```python
from build123d import *

# Parameters (mm, degrees)
SKETCH_1_R          = 3.25
EXTRUDE_1_DEPTH     = 2
SKETCH_1_3_W        = 8.5
SKETCH_1_3_H        = 1.5
EXTRUDE_2_DEPTH     = 1
SKETCH_2_W          = 4
SKETCH_2_H          = 1.5
EXTRUDE_3_DEPTH     = 6.5
CUT_EXTRUDE_1_DEPTH = 13
SKETCH_4_R          = 1.2
CUT_EXTRUDE_2_DEPTH = 13
SKETCH_5_W          = 0.419062678
SKETCH_5_H          = 3
CUT_EXTRUDE_3_DEPTH = 12
SKETCH_7_W          = 3.667600517
SKETCH_7_H          = 1.5
EXTRUDE_4_DEPTH     = 18
SKETCH_8_W          = 3.667600517
SKETCH_8_H          = 5.48261061
EXTRUDE_5_DEPTH     = 9
SKETCH_9_W          = 2.616581955
SKETCH_9_H          = 4.806747763
EXTRUDE_6_DEPTH     = 9
SKETCH_10_R         = 1.719166773
CUT_EXTRUDE_4_DEPTH = 11.421628998
CUT_EXTRUDE_5_DEPTH = 13
EXTRUDE_7_DEPTH     = 8.843258


with BuildPart() as part:
    # 草图1 → 凸台-拉伸1 (new body)
    with BuildSketch(Plane(origin=(0, 0, 0), x_dir=(1, 0, 0), z_dir=(0, 1, 0))):
        Polygon((-4.25, -4.25), (-4.25, -6), (4.25, -6), (4.25, -4.25), (4.25, 4.25), (4.25, 6), (-4.25, 6), (-4.25, 4.25), align=None)
        Circle(SKETCH_1_R, mode=Mode.SUBTRACT)
    extrude(amount=EXTRUDE_1_DEPTH)

    # 草图1<3> → 凸台-拉伸2 (add)
    with BuildSketch(Plane(origin=(0, 0, 0), x_dir=(1, 0, 0), z_dir=(0, 1, 0))):
        with Locations((0, -5.25)):
            Rectangle(SKETCH_1_3_W, SKETCH_1_3_H)
        with Locations((0, 5.25)):
            Rectangle(SKETCH_1_3_W, SKETCH_1_3_H)
    extrude(amount=-EXTRUDE_2_DEPTH)

    # 草图2 → 凸台-拉伸3 (add)
    with BuildSketch(Plane.XZ.offset(1)):
        with Locations((-1.830937322, -5.25)):
            Rectangle(SKETCH_2_W, SKETCH_2_H)
        with Locations((-1.830937322, 5.25)):
            Rectangle(SKETCH_2_W, SKETCH_2_H)
    extrude(amount=EXTRUDE_3_DEPTH)

    # 草图3 → 切除-拉伸1 (cut, through all)
    with BuildSketch(Plane(origin=(0, 0, -6), x_dir=(-1, 0, 0), z_dir=(0, 0, -1))):
        Polygon((-0.169062678, -4.270246896), (0.163336805, -7.5), (-0.169062678, -7.5), align=None)
    extrude(amount=-CUT_EXTRUDE_1_DEPTH, mode=Mode.SUBTRACT)

    # 草图4 → 切除-拉伸2 (cut, through all)
    with BuildSketch(Plane(origin=(0, 0, -6), x_dir=(-1, 0, 0), z_dir=(0, 0, -1))):
        with Locations((1.920905564, -6)):
            Circle(SKETCH_4_R)
    extrude(amount=-CUT_EXTRUDE_2_DEPTH, mode=Mode.SUBTRACT)

    # 草图5 → 切除-拉伸3 (cut)
    with BuildSketch(Plane(origin=(0, 0, -6), x_dir=(-1, 0, 0), z_dir=(0, 0, -1))):
        with Locations((4.040468661, 0.5)):
            Rectangle(SKETCH_5_W, SKETCH_5_H)
    extrude(amount=-CUT_EXTRUDE_3_DEPTH, mode=Mode.SUBTRACT)

    # 草图7 → 凸台-拉伸4 (add)
    with BuildSketch(Plane.XZ.offset(7.5)):
        with Locations((-1.997137064, 5.25)):
            Rectangle(SKETCH_7_W, SKETCH_7_H)
        with Locations((-1.997137064, -5.25)):
            Rectangle(SKETCH_7_W, SKETCH_7_H)
    extrude(amount=EXTRUDE_4_DEPTH)

    # 草图8 → 凸台-拉伸5 (add)
    with BuildSketch(Plane(origin=(0, 0, 4.5), x_dir=(-1, 0, 0), z_dir=(0, 0, -1))):
        with Locations((1.997137064, -22.758694695)):
            Rectangle(SKETCH_8_W, SKETCH_8_H)
    extrude(amount=EXTRUDE_5_DEPTH)

    # 草图9 → 凸台-拉伸6 (add)
    with BuildSketch(Plane(origin=(-0.163336805, 0, 0), x_dir=(0, 0, -1), z_dir=(1, 0, 0))):
        with Locations((3.113338021, -22.793424654)):
            Rectangle(SKETCH_9_W, SKETCH_9_H)
        with Locations((-3.113338021, -22.793424654)):
            Rectangle(SKETCH_9_W, SKETCH_9_H)
    extrude(amount=EXTRUDE_6_DEPTH)

    # 草图10 → 切除-拉伸4 (cut, through all)
    with BuildSketch(Plane(origin=(0, 0, -4.421628998), x_dir=(-1, 0, 0), z_dir=(0, 0, -1))):
        with Locations((-5.836663195, -22.894386417)):
            Circle(SKETCH_10_R)
    extrude(amount=-CUT_EXTRUDE_4_DEPTH, mode=Mode.SUBTRACT)

    # 草图11 → 切除-拉伸5 (cut, through all)
    with BuildSketch(Plane(origin=(0, 0, -6), x_dir=(-1, 0, 0), z_dir=(0, 0, -1))):
        Polygon((3.830937322, -22.440555736), (-3.067140817, -25.196798535), (0.381898253, -26.676483331), (3.830937322, -26.676483331), align=None)
    extrude(amount=-CUT_EXTRUDE_5_DEPTH, mode=Mode.SUBTRACT)

    # 草图13 → 凸台-拉伸7 (add)
    with BuildSketch(Plane(origin=(0, 0, -4.421628998), x_dir=(-1, 0, 0), z_dir=(0, 0, -1))):
        Polygon((-2.471529716, -20.390050772), (3.830937322, -16.84684298), (3.830937322, -20.390050772), align=None)
    extrude(amount=-EXTRUDE_7_DEPTH)


solid = part.part
```
Check sheet for the modelled part. Datum: model origin and axes. Units: mm. A direction names the side the tool comes from. Round coordinates to 2 decimals unless told otherwise and drop trailing zeros. Loops run counter-clockwise (first coordinate to the right, second up) from the corner with the lowest first, then second, coordinate; pieces in that order, holes last. Notation, with made-up numbers: M 27.5,60 L 43.5,60 A19 ccw 43.5,95 Z; hole C 16,-7 d5. An arc over 180 degrees is marked long. Answer as a JSON object with one key per item and string values.
1. Mould release check, pull along Z, two halves, no side actions. Record for faces 1 (the flat face through (0, -5.9, -5.3)), 2 (the flat face through (-2, -10, 4.5)), 3 (the flat face through (-2, -8, -6)): pulls with the +Z half, pulls with the -Z half, needs draft (parallel to the pull), parting line crosses it, or undercut.
Reply:
{"face 1": "needs draft", "face 2": "undercut", "face 3": "pulls with the -Z half"}
2. Section check B-B (x = 1.5). Record the boundary of the cut face in (y, z), plus the area to 3 significant figures.
Reply:
{"outline": "M -24.57,-4.42 L -19.84,-4.42 L -19.84,4.42 L -24.57,4.42 L -24.57,1.81 L -20.39,1.81 L -20.39,-1.81 L -24.57,-1.81 Z; M -1,-6 L 2,-6 L 2,-2.88 L 0,-2.88 L 0,-4.5 L -1,-4.5 Z; M -1,4.5 L 0,4.5 L 0,2.88 L 2,2.88 L 2,6 L -1,6 Z", "area": "42.2 mm²"}
3. Section check C-C (y = -0.5). Record the boundary of the cut face in (x, z).
Reply:
{"outline": "M -3.83,-6 L 4.25,-6 L 4.25,-4.5 L -3.83,-4.5 Z; M -3.83,4.5 L 4.25,4.5 L 4.25,6 L -3.83,6 Z"}
4. Access from +Z, -Z, +X, -X, +Y, -Y to the whole of each face (thin tool, end or side, straight path). Record for faces 4 (the flat face through (2, -22, -4.422)), 5 (the flat face through (0.169, -3, 5)), 6 (the cylindrical face through (-2.579, 0.986, 1.978)), 7 (the flat face through (-0.163, -22, 0)).
Reply:
{"face 4": "+X", "face 5": "+Z, -Z, +X, -Y", "face 6": "+Y", "face 7": "+X, -Y"}
5. Section check D-D (z = -4). Record the boundary of the cut face in (x, y), plus the area to 3 significant figures.
Reply:
{"outline": "M -3.83,-22.44 L 3.07,-25.2 L 8.84,-25.2 L 8.84,-20.39 L 2.47,-20.39 L -3.83,-16.85 Z; M -3.83,0 L 4.25,0 L 4.25,2 L -3.83,2 Z; hole C 5.84,-22.89 d3.44", "area": "69.4 mm²"}
6. Gauge pin test, flat ends, axial feed: P1, Ø2, axis at x = 5.84, y = -22.89, coming from the -Z side; P2, Ø4.5, axis at x = 5.84, y = -22.89, coming from the -Z side; P3, Ø1.5, axis at y = -19.5, z = -2.5, coming from the +X side; P4, Ø1.3, axis at x = 6, z = -3.5, coming from the +Y side. Record the tip position at first contact, or that the pin passes through.
Reply:
{"P1": "passes through", "P2": "stops at z = -4.42", "P3": "stops at x = 2.22", "P4": "stops at y = -20.39"}
7. Scan lines: line 1 (Z direction, x = -2.25, y = -13.5); line 2 (X direction, y = 1.55, z = 0); line 3 (Z direction, x = 0, y = 0.9). Record each from-to range of solid material in increasing order.
Reply:
{"line 1": "z = -6 to -4.5, 4.5 to 6", "line 2": "x = -3.83 to -3.25, 3.25 to 4.25", "line 3": "z = -6 to -3.25, 3.25 to 6"}
8. Section check A-A (z = -2.75). Record the boundary of the cut face in (x, y).
Reply:
{"outline": "M -3.83,-22.44 L 3.07,-25.2 L 8.84,-25.2 L 8.84,-20.39 L 2.47,-20.39 L -3.83,-16.85 Z; M -3.83,0 L -1.73,0 L -1.73,2 L -3.83,2 Z; M 1.73,0 L 4.25,0 L 4.25,2 L 1.73,2 Z; hole C 5.84,-22.89 d3.44"}
